Can you work these out from the model? Positions are in its coordinate system, mm. A direction names the side the tool comes from. Give positions to 0.01 mm unless a question says otherwise; leave off trailing zeros. Loops run counter-clockwise (first coordinate to the right, second up) from the corner with the lowest first, then second, coordinate; pieces in that order, holes last. Notation, with made-up numbers: (22, -6) - (53, -6) arc R21 ccw to (53, 5) - close; hole circle Ø4 at (83.25, 41). An arc over 180 degrees is marked (long way). Write item = value, one per line.
from build123d import *
from build123d.topology import SkipClean

# Parameters (mm, degrees)
SKETCH_1_R      = 12.5
SKETCH_1_R_2    = 11.05
EXTRUDE_1_DEPTH = 5
EXTRUDE_2_DEPTH = 20
SKETCH_3_R      = 12.5
SKETCH_3_R_2    = 11.05
EXTRUDE_3_DEPTH = 5
SKETCH_4_R      = 1.55
EXTRUDE_5_DEPTH = 3
EXTRUDE_START   = -30
EXTRUDE_7_DEPTH = 30
SKETCH_7_W      = 12
SKETCH_7_H      = 12
SKETCH_7_R      = 5.1
EXTRUDE_8_DEPTH = 10


with BuildPart() as part:
    # 草图1 → 凸台-拉伸1 (new body)
    with BuildSketch(Plane(origin=(0, 0, 0), x_dir=(1, 0, 0), z_dir=(0, 1, 0))):
        with Locations(Location((0, 0, 0), (0, 0, 270))):
            Circle(SKETCH_1_R)
        with Locations(Location((0, 0, 0), (0, 0, 270))):
            Circle(SKETCH_1_R_2, mode=Mode.SUBTRACT)
    extrude(amount=EXTRUDE_1_DEPTH)

    # 草图2 → 凸台-拉伸2 (add)
    with SkipClean():  # the faces are left unmerged after this step: merging them gives an invalid solid
        with BuildSketch(Plane(origin=(0, 5, 0), x_dir=(1, 0, 0), z_dir=(0, 1, 0))):
            with BuildLine():
                Line((-10.825318, 6.25), (-9.569581, 5.525))
                ThreePointArc((-9.569581, 5.525), (-7.81353, 7.81353), (-5.525, 9.569581))
                Line((-5.525, 9.569581), (-6.25, 10.825318))
                ThreePointArc((-6.25, 10.825318), (-8.838835, 8.838835), (-10.825318, 6.25))
            make_face()
            with BuildLine():
                Line((0, 12.5), (0, 11.05))
                ThreePointArc((0, 11.05), (2.85995, 10.67348), (5.525, 9.569581))
                Line((5.525, 9.569581), (6.25, 10.825318))
                ThreePointArc((6.25, 10.825318), (3.235238, 12.074073), (0, 12.5))
            make_face()
            with BuildLine():
                Line((10.825318, 6.25), (9.569581, 5.525))
                ThreePointArc((9.569581, 5.525), (10.67348, 2.85995), (11.05, 0))
                Line((11.05, 0), (12.5, 0))
                ThreePointArc((12.5, 0), (12.074073, 3.235238), (10.825318, 6.25))
            make_face()
            with BuildLine():
                Line((10.825318, -6.25), (9.569581, -5.525))
                ThreePointArc((9.569581, -5.525), (7.81353, -7.81353), (5.525, -9.569581))
                Line((5.525, -9.569581), (6.25, -10.825318))
                ThreePointArc((6.25, -10.825318), (8.838835, -8.838835), (10.825318, -6.25))
            make_face()
            with BuildLine():
                Line((0, -12.5), (0, -11.05))
                ThreePointArc((0, -11.05), (-2.85995, -10.67348), (-5.525, -9.569581))
                Line((-5.525, -9.569581), (-6.25, -10.825318))
                ThreePointArc((-6.25, -10.825318), (-3.235238, -12.074073), (0, -12.5))
            make_face()
            with BuildLine():
                Line((-10.825318, -6.25), (-9.569581, -5.525))
                ThreePointArc((-9.569581, -5.525), (-10.67348, -2.85995), (-11.05, 0))
                Line((-11.05, 0), (-12.5, 0))
                ThreePointArc((-12.5, 0), (-12.074073, -3.235238), (-10.825318, -6.25))
            make_face()
        extrude(amount=EXTRUDE_2_DEPTH)

    # 草图3 → 凸台-拉伸3 (add)
    with SkipClean():  # the faces are left unmerged after this step: merging them gives an invalid solid
        with BuildSketch(Plane(origin=(0, 25, 0), x_dir=(1, 0, 0), z_dir=(0, 1, 0))):
            with Locations(Location((0, 0, 0), (0, 0, 270))):
                Circle(SKETCH_3_R)
            with Locations(Location((0, 0, 0), (0, 0, 270))):
                Circle(SKETCH_3_R_2, mode=Mode.SUBTRACT)
        extrude(amount=EXTRUDE_3_DEPTH)

    # 草图4 → 凸台-拉伸5 (add)
    # profile 1 of 2: a face of its own
    with SkipClean():  # the faces are left unmerged after this step: merging them gives an invalid solid
        with BuildSketch(Plane(origin=(0, 30, 0), x_dir=(1, 0, 0), z_dir=(0, 1, 0))):
            with BuildLine():
                Line((-7, -3), (-7, 3))
                Line((-7, 3), (-11.489313, 4.923991))
                ThreePointArc((-11.489313, 4.923991), (-12.5, 0), (-11.489313, -4.923991))
                Line((-11.489313, -4.923991), (-7, -3))
            make_face()
            with Locations(Location((-9.5, 0, 0), (0, 0, 179.999298))):
                Circle(SKETCH_4_R, mode=Mode.SUBTRACT)
        # profile 2 of 2: a face of its own
        with BuildSketch(Plane(origin=(0, 30, 0), x_dir=(1, 0, 0), z_dir=(0, 1, 0))):
            with BuildLine():
                Line((7, -3), (11.489313, -4.923991))
                ThreePointArc((11.489313, -4.923991), (12.5, 0), (11.489313, 4.923991))
                Line((11.489313, 4.923991), (7, 3))
                Line((7, 3), (7, -3))
            make_face()
            with Locations((9.5, 0)):
                Circle(SKETCH_4_R, mode=Mode.SUBTRACT)
        extrude(amount=EXTRUDE_5_DEPTH)

    # 凸台-拉伸7: read off the stored shape, not the designer's step
    # 凸台-拉伸7 outline → 凸台-拉伸7 (add)
    with BuildSketch(Plane(origin=(0, 30, 0), x_dir=(1, 0, 0), z_dir=(0, 1, 0)).offset(EXTRUDE_START)):
        with BuildLine():
            ThreePointArc((-5.525, -9.569581), (-6.321565, -9.06313), (-7.072, -8.490543))
            Line((-7.072, -8.490543), (-8, -9.604686))
            Line((-8, -9.604686), (-8, -12.5))
            Line((-8, -12.5), (0, -12.5))
            ThreePointArc((0, -12.5), (-3.235238, -12.074073), (-6.25, -10.825318))
            Line((-6.25, -10.825318), (-5.525, -9.569581))
        make_face()
        with BuildLine():
            ThreePointArc((5.525, -9.569581), (2.85995, -10.67348), (0, -11.05))
            Line((0, -11.05), (0, -12.5))
            Line((0, -12.5), (8, -12.5))
            Line((8, -12.5), (8, -9.604686))
            ThreePointArc((8, -9.604686), (7.151092, -10.252409), (6.25, -10.825318))
            Line((6.25, -10.825318), (5.525, -9.569581))
        make_face()
    extrude(amount=EXTRUDE_7_DEPTH)

    # 草图7 → 凸台-拉伸8 (add)
    with BuildSketch(Plane.XY.offset(12.5)):
        with Locations((0, 15)):
            Rectangle(SKETCH_7_W, SKETCH_7_H)
        with Locations((0, 15)):
            Circle(SKETCH_7_R, mode=Mode.SUBTRACT)
    extrude(amount=EXTRUDE_8_DEPTH)


solid = part.part
Q1. We'd pull the mould along X, two halves only. Please class faces 6 (the flat face through (1.9, 0, 11.1)), 7 (the flat face through (-7.53, 14.86, 9.04)), 8 (the flat face through (-7, 31, 0)), 9 (the flat face through (8, 15, 11)): released by +X, released by -X, zero draft, split by the parting line, or undercut.
Output:
face_6 = zero draft
face_7 = released by -X
face_8 = undercut
face_9 = released by +X
Q2. I need wall thicknesses on L1, parallel to X at y = 30.95, z = 0; L2, parallel to Z at x = 0, y = 28; L3, parallel to X at y = 25.5, z = 7.5. Which ranges of each line are inside material? Lowest first, please.
Output:
L1 = -12.5 to -11.05, -7.95 to -7, 7 to 7.95, 11.05 to 12.5
L2 = -12.5 to -11.05, 11.05 to 12.5
L3 = -10 to -8.11, 8.11 to 10
Q3. For pin 1 (5 mm diameter, centred on x = -1, y = 15.5, fed in from +Z); pin 2 (1.5 mm diameter, centred on x = 3, z = 13.5, fed in from -Y); pin 3 (2 mm diameter, centred on y = 20, z = -8, fed in from +X); pin 4 (12 mm diameter, centred on x = 3.5, z = 0, fed in from +Y), each with a flat end and sliding along its axis, tell me the tip position at first contact or that it passes through.
Output:
pin_1 = 12.5
pin_2 = 9
pin_3 = -6.41
pin_4 = 33
Q4. Imagine slicing it at D-D, the plane x = 3. Write out the boundary of the cut face in (y, z), then the cut area to 3 significant figures.
Output:
outline = (0, -12.13) - (30, -12.13) - (30, -10.63) - (0, -10.63) - close; (0, 10.63) - (30, 10.63) - (30, 12.5) - (21, 12.5) - (21, 22.5) - (19.12, 22.5) - (19.12, 12.5) - (10.88, 12.5) - (10.88, 22.5) - (9, 22.5) - (9, 12.5) - (0, 12.5) - close
area = 138 mm2
Q5. Which directions (+Z, -Z, +X, -X, +Y, -Y) give clear straight access to the entire face, cutting with the end or side of a thin tool? Please do faces 1 (the cylindrical face through (2.821, 14.86, -10.684)), 2 (the cylindrical face through (-1, 10, 17)), 3 (the flat face through (-3, 25, -11)), 4 (the flat face through (9.213, 31.479, 3.949)), 5 (the flat face through (9.276, 31.479, -3.975)).
Output:
face_1 = +Y, -Y
face_2 = +Z
face_3 = -Z
face_4 = +Z, +Y
face_5 = -Z, +Y
Q6. Imagine slicing it at C-C, the plane x = -4.5. Write out the boundary of the cut face in (y, z).
Output:
outline = (0, -11.66) - (5, -11.66) - (5, -10.09) - (0, -10.09) - close; (0, 10.09) - (30, 10.09) - (30, 12.5) - (21, 12.5) - (21, 22.5) - (17.4, 22.5) - (17.4, 12.5) - (12.6, 12.5) - (12.6, 22.5) - (9, 22.5) - (9, 12.5) - (0, 12.5) - close; (25, -11.66) - (30, -11.66) - (30, -10.09) - (25, -10.09) - close
Q7. Imagine slicing it at B-B, the plane z = -8.5. Write out the boundary of the cut face in (x, y).
Output:
outline = (-9.17, 0) - (-7.06, 0) - (-7.06, 30) - (-9.17, 30) - close; (7.06, 0) - (9.17, 0) - (9.17, 5) - (7.06, 5) - close; (7.06, 25) - (9.17, 25) - (9.17, 30) - (7.06, 30) - close
Q8. Imagine slicing it at A-A, the plane y = 15. Give the number of separate pieces and of enclosed holes in the cut face, then the cut area to 3 significant figures.
Output:
separate_pieces = 5
enclosed_holes = 0
area = 98.1 mm2
